```python
from build123d import *

# Parameters (mm, degrees)
SKETCH1_W           = 78.2
SKETCH1_H           = 58
BOSS_EXTRUDE1_DEPTH = 3
SKETCH2_R           = 1.5
CUT_EXTRUDE1_DEPTH  = 3
SKETCH3_R           = 1.5
CUT_EXTRUDE2_DEPTH  = 3


with BuildPart() as part:
    # Sketch1 → Boss-Extrude1 (new body)
    with BuildSketch(Plane(origin=(0, 0, 0), x_dir=(1, 0, 0), z_dir=(0, 1, 0))):
        Rectangle(SKETCH1_W, SKETCH1_H)
    extrude(amount=BOSS_EXTRUDE1_DEPTH)

    # Sketch2 → Cut-Extrude1 (cut)
    with BuildSketch(Plane(origin=(0, 3, 0), x_dir=(1, 0, 0), z_dir=(0, 1, 0))):
        with Locations(Location((-34.6, 24.5, 0), (0, 0, 270))):
            Circle(SKETCH2_R)
        with Locations(Location((-34.6, -24.5, 0), (0, 0, 270))):
            Circle(SKETCH2_R)
    extrude(amount=-CUT_EXTRUDE1_DEPTH, mode=Mode.SUBTRACT)

    # Sketch3 → Cut-Extrude2 (cut)
    with BuildSketch(Plane(origin=(0, 3, 0), x_dir=(1, 0, 0), z_dir=(0, 1, 0))):
        with Locations(Location((27.1, 20, 0), (0, 0, 270))):
            Circle(SKETCH3_R)
        with Locations(Location((27.1, -19, 0), (0, 0, 270))):
            Circle(SKETCH3_R)
    extrude(amount=-CUT_EXTRUDE2_DEPTH, mode=Mode.SUBTRACT)


solid = part.part
```
Work out the finished part from the listing and answer in its coordinate system (mm). Give positions to 0.01 mm unless a question says otherwise; leave off trailing zeros. Loops run counter-clockwise (first coordinate to the right, second up) from the corner with the lowest first, then second, coordinate; pieces in that order, holes last. Notation, with made-up numbers: M 57.25,14 L 70.25,14 A30 ccw 70.25,39 Z; hole C -37.75,54 d1. An arc over 180 degrees is marked long. One line per item, written item: value. Start each with the question number.
1. This flat-tipped pin is pushed along its axis until it touches: P1, Ø1.8, axis at x = -34.6, z = 24.5, coming from the -Y side. Where does it stop, or does it pass through?
2. Find the intervals of material crossed by probe 1 along X at (y, z) = (1.5, -20); probe 2 along X at (y, z) = (2.8, -24.5), in increasing order.
3. Find section A-A (z = 24.5). Give the vertices of the cut face in (x, y), and give its area (3 significant figures).
Reported:
1. P1: passes through
2. probe 1: x = -39.1 to 25.6, 28.6 to 39.1
2. probe 2: x = -39.1 to -36.1, -33.1 to 39.1
3. outline: M -39.1,0 L -36.1,0 L -36.1,3 L -39.1,3 Z; M -33.1,0 L 39.1,0 L 39.1,3 L -33.1,3 Z
3. area: 226 mm²
